```python
from build123d import *

# Parameters (mm, degrees)
F0_R      = 10
F1_DEPTH  = 35
F0_R_2    = 20
F1_FACE_R = 10
F2_DEPTH  = 100
F3_R      = 10
F4_DEPTH  = 25
F5_R      = 7
F6_DEPTH  = 50
F7_R      = 7
F8_DEPTH  = 50


with BuildPart() as f1:
    # F0 (on Top) → F1 (new body)
    with BuildSketch(Plane.XY):
        Circle(F0_R)
    extrude(amount=-F1_DEPTH)

    # F0 (on Top) + F1_face (on face) → F2 (join)
    with BuildSketch(Plane.XY):
        Circle(F0_R_2)
        Circle(F0_R, mode=Mode.SUBTRACT)
    with BuildSketch(Plane.XY):
        Circle(F1_FACE_R)
    extrude(amount=F2_DEPTH)

    # F3 (on face) → F4 (join)
    with BuildSketch(Plane.XY.offset(100)):
        Circle(F3_R)
    extrude(amount=F4_DEPTH)

    # F5 (on face) → F6 (cut)
    with BuildSketch(Plane.XY.offset(125)):
        Circle(F5_R)
    extrude(amount=-F6_DEPTH, mode=Mode.SUBTRACT)

    # F7 (on face) → F8 (cut)
    with BuildSketch(Plane(origin=(0, 0, -35), x_dir=(1, 0, 0), z_dir=(0, 0, -1))):
        Circle(F7_R)
    extrude(amount=-F8_DEPTH, mode=Mode.SUBTRACT)


solid = f1.part
```
Geometry: final body of the model. Coordinates: model frame, mm. A direction names the side the tool comes from. Round coordinates to 2 decimals unless told otherwise and drop trailing zeros. Write each loop counter-clockwise with the first axis right and the second up, starting at its lowest first coordinate (ties: lowest second). Pieces come first, ordered by that corner, then holes.
Item 1: Pin query (flat end, axial travel): P1, Ø7, axis at x = -1.5, y = 2, coming from the +Z side; P2, Ø2, axis at y = 11, z = 42.5, coming from the +X side; P3, Ø3, axis at y = 12, z = 0.5, coming from the +X side. Return the tip coordinate at first contact, or that it passes through.
Item 2: Section query D-D (z = 34.5). Return loops of the section in (x, y).
Item 3: Mould query, pull axis Y, two halves, no side actions, for faces 1 (the face through (0, 0, 75)), 2 (the face through (-2.17, -9.76, -17.26)), 3 (the face through (-7, -2, -35)). Classes: +Y half, -Y half, draft (parallel to the pull), parting line (faces both ways), or undercut.
Item 4: Section query A-A (x = 0). Return loops of the section in (y, z), plus the area to 3 significant figures.
Item 5: Material intervals for L1, parallel to Y at x = 0, z = -13; L2, parallel to Z at x = -5.5, y = 9; L3, parallel to X at y = -4.5, z = 86, sorted ascending.
Item 6: Section query C-C (z = 107). Return loops of the section in (x, y).
Item 7: Set-up query: faces 4 (the face through (6.466, 2.681, -10.35)), 5 (the face through (-2.17, -9.76, 112.32)), 6 (the face through (-4.336, -19.524, 49.3)). Return all of +Z, -Z, +X, -X, +Y, -Y with unobstructed straight access to the full face (end or side cutting, diameter ignored); none if empty.
Completed:
1. P1: stops at z = 75
1. P2: stops at x = 17.32
1. P3: stops at x = 17.02
2. outline: circle Ø40 at (0, 0)
3. face 1: undercut
3. face 2: parting line
3. face 3: draft
4. outline: (-20, 0) - (-10, 0) - (-10, -35) - (-7, -35) - (-7, 15) - (7, 15) - (7, -35) - (10, -35) - (10, 0) - (20, 0) - (20, 100) - (10, 100) - (10, 125) - (7, 125) - (7, 75) - (-7, 75) - (-7, 125) - (-10, 125) - (-10, 100) - (-20, 100) - close
4. area: 3,800 mm2
5. L1: y = -10 to -7, 7 to 10
5. L2: z = 0 to 100
5. L3: x = -19.49 to -5.36, 5.36 to 19.49
6. outline: circle Ø20 at (0, 0); hole circle Ø14 at (0, 0)
7. face 4: -Z
7. face 5: +Z
7. face 6: +Z, -Z
